Autodesk Inventor part; units mm, degrees
ref_plane "YZ Plane" through (0, 0, 0) normal (1, 0, 0) x (0, 1, 0)
ref_plane "XZ Plane" through (0, 0, 0) normal (0, 1, 0) x (-1, 0, 0)
ref_plane "XY Plane" through (0, 0, 0) normal (0, 0, 1) x (1, 0, 0)
sketch "Skizze1" plane through (0, 0, 0) normal (0, 0, 1) x (1, 0, 0)
  line L0 (0, 0) -> (0, 200)
  line L1 (0, 200) -> (120, 200)
  line L2 (120, 200) -> (120, 90)
  line L3 (120, 90) -> (200, 90)
  line L4 (200, 90) -> (200, 200)
  line L5 (200, 200) -> (320, 200)
  line L6 (320, 200) -> (320, 0)
  line L7 (320, 0) -> (0, 0)
  line L8 (5, 60) -> (15, 60)
  line L9 (15, 60) -> (15, 140)
  line L10 (15, 140) -> (5, 140)
  line L11 (5, 140) -> (5, 60)
  line L12 (70, 140) -> (95, 140)
  line L13 (95, 140) -> (95, 60)
  line L14 (95, 60) -> (70, 60)
  line L15 (70, 60) -> (70, 140)
  line L16 (250, 140) -> (225, 140)
  line L17 (225, 140) -> (225, 60)
  line L18 (225, 60) -> (250, 60)
  line L19 (250, 60) -> (250, 140)
  line L20 (315, 140) -> (305, 140)
  line L21 (305, 140) -> (305, 60)
  line L22 (305, 60) -> (315, 60)
  line L23 (315, 60) -> (315, 140)
  dimension "d0" = 320
  dimension "d1" = 200
  dimension "d4" = 110
  dimension "d5" = 80
  dimension "d6" = 10
  dimension "d7" = 25
  dimension "d8" = 80
  dimension "d9" = 25
  dimension "d10" = 80
  dimension "d11" = 10
  dimension "d12" = 5
  dimension "d13" = 55
  dimension "d14" = 55
  dimension "d15" = 5
  dimension "d16" = 60
  dimension "d17" = 60
  dimension "d18" = 60
  dimension "d21" = 105
  dimension "d22" = 105
extrude "Extrusion1" add sketch "Skizze1" along normal blind 6
hole "Bohrung1" at (38, 105, 6) direction (0, 0, -1) diameter 5 depth 8 tip angle 118
hole "Bohrung2" at (38, 95, 6) direction (0, 0, -1) diameter 5 depth 8 tip angle 118
hole "Bohrung5" at (282, 105, 6) direction (0, 0, -1) diameter 5 depth 8 tip angle 118
hole "Bohrung6" at (282, 95, 6) direction (0, 0, -1) diameter 5 depth 8 tip angle 118
properties part number "FahrwerkbasisBsp"
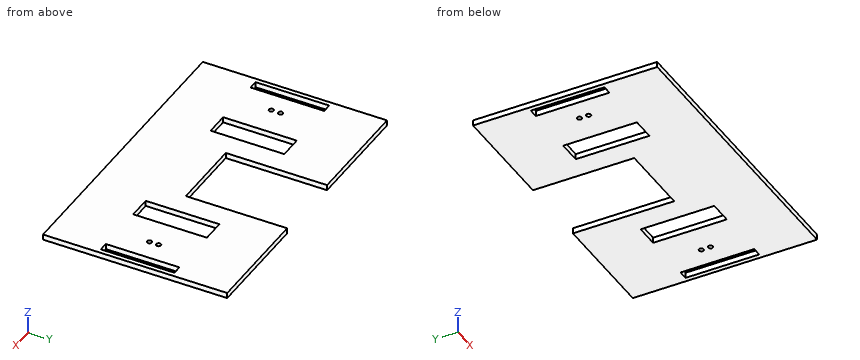
Design review of the part built by this model. Coordinates are the model's own, in mm. Round coordinates to 2 decimals unless told otherwise and drop trailing zeros. Loops run counter-clockwise (first coordinate to the right, second up) from the corner with the lowest first, then second, coordinate; pieces in that order, holes last. Notation, with made-up numbers: (69.25, 44) - (112.25, 44) arc R8 ccw to (112.25, 53) - close; hole circle Ø2 at (58, 81.25). An arc over 180 degrees is marked (long way). One line per item, written item: value. Start each with the question number.
1) To check wall thickness, follow L1, parallel to Y at x = 282, z = 1.55; L2, parallel to X at y = 160, z = 4.3; L3, parallel to Y at x = 75.5, z = 2. State the ranges of each line that lie inside material, in increasing order. Write a range as from..to.
2) Insertion check: pin 1 Ø1.8 at (x, z) = (173.5, 2) entering from +Y; pin 2 Ø4 at (x, y) = (282, 95) entering from -Z. Each pin has a flat end and moves straight along its axis. Give the tip position at first contact, or say it passes through.
3) Consider section B-B on z = 3.3. Give the number of separate pieces and of enclosed holes in the cut face, then the cut area to 3 significant figures.
4) Consider section C-C on y = 69. Give the boundary of the cut face in (x, z).
5) Consider section A-A on y = 121. Give the boundary of the cut face in (x, z).
Reported:
1. L1: y = 0..92.5, 97.5..102.5, 107.5..200
1. L2: x = 0..120, 200..320
1. L3: y = 0..60, 140..200
2. pin 1: stops at y = 90
2. pin 2: passes through
3. separate pieces: 1
3. enclosed holes: 8
3. area: 49,500 mm^2
4. outline: (0, 0) - (5, 0) - (5, 6) - (0, 6) - close; (15, 0) - (70, 0) - (70, 6) - (15, 6) - close; (95, 0) - (225, 0) - (225, 6) - (95, 6) - close; (250, 0) - (305, 0) - (305, 6) - (250, 6) - close; (315, 0) - (320, 0) - (320, 6) - (315, 6) - close
5. outline: (0, 0) - (5, 0) - (5, 6) - (0, 6) - close; (15, 0) - (70, 0) - (70, 6) - (15, 6) - close; (95, 0) - (120, 0) - (120, 6) - (95, 6) - close; (200, 0) - (225, 0) - (225, 6) - (200, 6) - close; (250, 0) - (305, 0) - (305, 6) - (250, 6) - close; (315, 0) - (320, 0) - (320, 6) - (315, 6) - close
